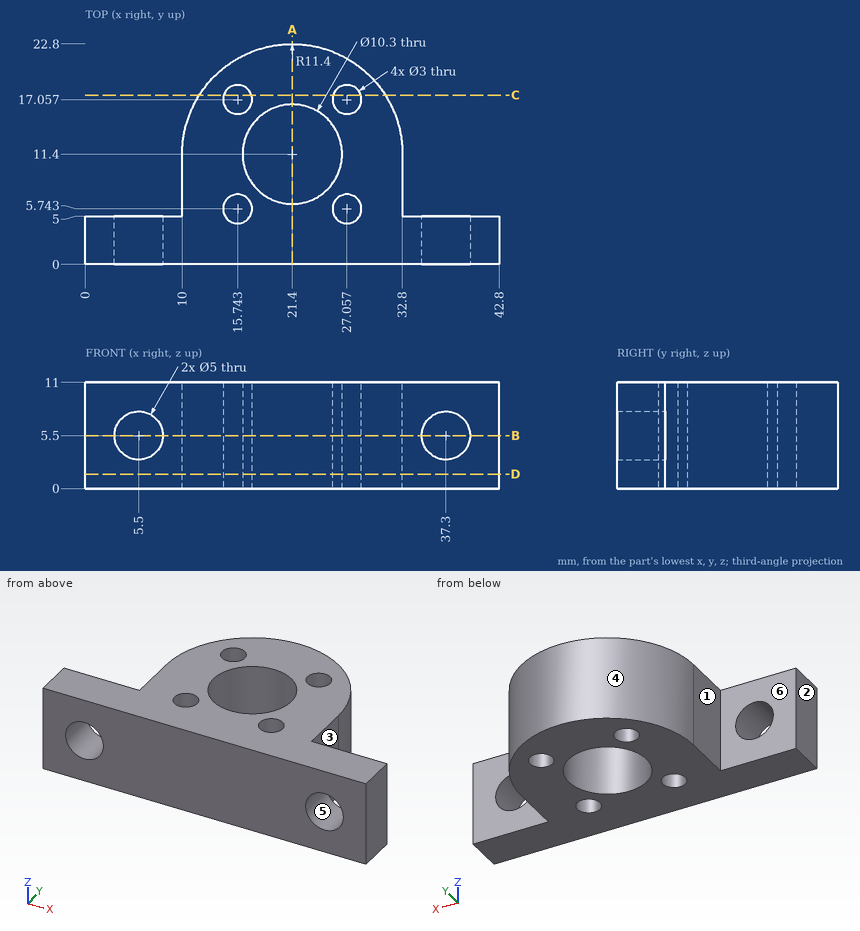
Geometry check sheet. Reference: drawing and pictorial views, mm from the part's lowest x, y, z. A direction names the side the tool comes from. Coordinates: 2 decimals unless noted, no trailing zeros. Order: outer loops, then holes, each group sorted by start corner. A loop starts at its lowest first (then second) coordinate and runs counter-clockwise, first axis right, second up. Notation, with made-up numbers: (-31.75, 20) -> (24.25, 20) arc R18 ccw to (24.25, 28) -> close; hole circle Ø1 at (63, 67.25). An arc over 180 degrees is marked (long way). Put each result on its own line as item: value. Start each with the question number.
1) Material ranges on L1, parallel to Y at x = 21.4, z = 4.25; L2, parallel to Y at x = 15, z = 1.5; L3, parallel to Y at x = 15.5, z = 9 (1 decimal), recorded low to high.
2) Go/stop test with flat-tipped pins: pin 1 (2.5 mm diameter, centred on x = 27.06, y = 5.74, fed in from -Z); pin 2 (2 mm diameter, centred on y = 10.5, z = 2, fed in from -X); pin 3 (1.5 mm diameter, centred on y = 14.5, z = 8.5, fed in from +X) (3 decimals); pin 4 (5 mm diameter, centred on y = 8.5, z = 7.5, fed in from +X). Record where each tip stops, or that it passes through.
3) Cross-section at C-C (y = 17.5). Enter the section's corners in (x, z).
4) Tool access check on the marked faces 1, 2 and 3. Record the directions out of +Z, -Z, +X, -X, +Y, -Y that give a thin tool (end or side, any length) a straight path to the whole face; none if there is none.
5) Cross-section at A-A (x = 21.4). Enter the section's corners in (y, z).
6) Cross-section at B-B (z = 5.5). Enter the section's corners in (x, y).
7) Cross-section at D-D (z = 1.5). Enter the section's corners in (x, y).
8) Release check for a two-part mould opening along X. For the marked faces 4, 5 and 6 record: pulls with the +X half, pulls with the -X half, needs draft (parallel to the pull), parting line crosses it, or undercut.
Geometry check:
1. L1: y = 0 to 6.25, 16.55 to 22.8
1. L2: y = 0 to 4.44, 7.05 to 15.75, 18.36 to 20.83
1. L3: y = 0 to 4.3, 7.2 to 15.6, 18.5 to 21.2
2. pin 1: passes through
2. pin 2: stops at x = 10
2. pin 3: stops at x = 32.555
2. pin 4: stops at x = 32.8
3. outline: (11.77, 0) -> (14.31, 0) -> (14.31, 11) -> (11.77, 11) -> close; (17.18, 0) -> (25.62, 0) -> (25.62, 11) -> (17.18, 11) -> close; (28.49, 0) -> (31.03, 0) -> (31.03, 11) -> (28.49, 11) -> close
4. face 1: +Z, -Z, -X, +Y
4. face 2: +Z, -Z, -X, +Y, -Y
4. face 3: +Z, -Z, +X, +Y
5. outline: (0, 0) -> (6.25, 0) -> (6.25, 11) -> (0, 11) -> close; (16.55, 0) -> (22.8, 0) -> (22.8, 11) -> (16.55, 11) -> close
6. outline: (0, 0) -> (3, 0) -> (3, 5) -> (0, 5) -> close; (8, 0) -> (34.8, 0) -> (34.8, 5) -> (32.8, 5) -> (32.8, 11.4) arc R11.4 ccw to (10, 11.4) -> (10, 5) -> (8, 5) -> close; (39.8, 0) -> (42.8, 0) -> (42.8, 5) -> (39.8, 5) -> close; hole circle Ø3 at (15.74, 5.74); hole circle Ø3 at (15.74, 17.06); hole circle Ø10.3 at (21.4, 11.4); hole circle Ø3 at (27.06, 5.74); hole circle Ø3 at (27.06, 17.06)
7. outline: (0, 0) -> (42.8, 0) -> (42.8, 5) -> (32.8, 5) -> (32.8, 11.4) arc R11.4 ccw to (10, 11.4) -> (10, 5) -> (0, 5) -> close; hole circle Ø3 at (15.74, 5.74); hole circle Ø3 at (15.74, 17.06); hole circle Ø10.3 at (21.4, 11.4); hole circle Ø3 at (27.06, 5.74); hole circle Ø3 at (27.06, 17.06)
8. face 4: parting line crosses it
8. face 5: undercut
8. face 6: needs draft
